The listing builds one solid part. Answer for the finished solid, in the listing's coordinates (mm). Give positions to 0.01 mm unless a question says otherwise; leave off trailing zeros. Loops run counter-clockwise (first coordinate to the right, second up) from the corner with the lowest first, then second, coordinate; pieces in that order, holes last. Notation, with made-up numbers: M 2,36.25 L 22,36.25 A21 cw 22,49.25 Z; hole C -27.75,80 d5. An arc over 180 degrees is marked long. Use one line per item in the form item = value. Start each with the question number.
1. Straight lines are drawn through the part: line 1 (X direction, y = -0.95, z = 7); line 2 (Z direction, x = -24.5, y = -0.9); line 3 (Z direction, x = -24, y = -0.8). For each, find the intervals that lie inside material, in ascending order. Write a range as from..to.
2. The part is cut by section A-A (z = 37). Write down the section's boundary in (x, y), and give its area (3 significant figures).
3. The mould has two halves that part along Z. Classify faces 1 (the face through (0, -1, -30)), 2 (the face through (-23.265, -0.986, 6.772)), 3 (the face through (32, -1, 23)): released by +Z, released by -Z, zero draft, split by the parting line, or undercut.
4. The part is cut by section B-B (z = 67). Write down the section's boundary in (x, y).
from build123d import *

# Parameters (mm, degrees)
SKETCH1_W          = 64
SKETCH1_H          = 2
BASE_FLANGE1_DEPTH = 74
SKETCH2_R          = 1.75
CUT_EXTRUDE1_DEPTH = 10
CHAMFER1_SIZE      = 2
SKETCH8_W          = 64
SKETCH8_H          = 30
TAB1_DEPTH         = 2
CHAMFER2_SIZE      = 2
CUT_EXTRUDE2_REACH = 82.647
SKETCH9_R          = 2.25


# Sheet-metal steps are written as plain solids
with BuildPart() as part:
    # Sketch1 → Base-Flange1 (new body)
    with BuildSketch(Plane.XY):
        with Locations((0, -1)):
            Rectangle(SKETCH1_W, SKETCH1_H)
    extrude(amount=BASE_FLANGE1_DEPTH)

    # Sketch2 → Cut-Extrude1 (cut)
    with BuildSketch(Plane(origin=(0, 0, 0), x_dir=(1, 0, 0), z_dir=(0, 1, 0))):
        with Locations(Location((-25, -7, 0), (0, 0, 270))):
            Circle(SKETCH2_R)
        with Locations(Location((-25, -67, 0), (0, 0, 270))):
            Circle(SKETCH2_R)
        with Locations(Location((25, -67, 0), (0, 0, 270))):
            Circle(SKETCH2_R)
        with Locations(Location((25, -7, 0), (0, 0, 270))):
            Circle(SKETCH2_R)
    extrude(amount=-CUT_EXTRUDE1_DEPTH, mode=Mode.SUBTRACT)

    # Chamfer1
    chamfer1_edges = [part.edges().sort_by_distance(p)[0] for p in [
        (-32, -1, 74),
        (32, -1, 74),
    ]]
    chamfer(chamfer1_edges, length=CHAMFER1_SIZE)

    # Sketch8 → Tab1 (add)
    with BuildSketch(Plane(origin=(0, 0, 0), x_dir=(1, 0, 0), z_dir=(0, 1, 0))):
        with Locations((0, 15)):
            Rectangle(SKETCH8_W, SKETCH8_H)
    extrude(amount=-TAB1_DEPTH)

    # Chamfer2
    chamfer2_edges = [part.edges().sort_by_distance(p)[0] for p in [
        (-32, -1, -30),
        (32, -1, -30),
    ]]
    chamfer(chamfer2_edges, length=CHAMFER2_SIZE)

    # Sketch9 → Cut-Extrude2 (cut, up to next)
    with BuildSketch(Plane(origin=(0, 0, 0), x_dir=(1, 0, 0), z_dir=(0, 1, 0)), mode=Mode.PRIVATE) as cut_extrude2_sk1:
        with Locations(Location((-25.25, -37, 0), (0, 0, 270))):
            Circle(SKETCH9_R)
    cut_extrude2_tool1 = extrude(cut_extrude2_sk1.sketch, amount=-CUT_EXTRUDE2_REACH, mode=Mode.PRIVATE) & part.part
    # Sketch9 → Cut-Extrude2 (cut, up to next)
    with BuildSketch(Plane(origin=(0, 0, 0), x_dir=(1, 0, 0), z_dir=(0, 1, 0)), mode=Mode.PRIVATE) as cut_extrude2_sk2:
        with Locations(Location((25.25, -37, 0), (0, 0, 270))):
            Circle(SKETCH9_R)
    cut_extrude2_tool2 = extrude(cut_extrude2_sk2.sketch, amount=-CUT_EXTRUDE2_REACH, mode=Mode.PRIVATE) & part.part
    add(cut_extrude2_tool1.solids().sort_by_distance((-25.25, 0, 37))[0], mode=Mode.SUBTRACT)
    add(cut_extrude2_tool2.solids().sort_by_distance((25.25, 0, 37))[0], mode=Mode.SUBTRACT)


solid = part.part
Derived:
q1.line_1 = -32..-26.75, -23.25..23.25, 26.75..32
q1.line_2 = -30..5.32, 8.68..34.88, 39.12..65.32, 68.68..74
q1.line_3 = -30..5.56, 8.44..35.13, 38.87..65.56, 68.44..74
q2.outline = M -32,-2 L -27.5,-2 L -27.5,0 L -32,0 Z; M -23,-2 L 23,-2 L 23,0 L -23,0 Z; M 27.5,-2 L 32,-2 L 32,0 L 27.5,0 Z
q2.area = 110 mm2
q3.face_1 = released by -Z
q3.face_2 = undercut
q3.face_3 = zero draft
q4.outline = M -32,-2 L -26.75,-2 L -26.75,0 L -32,0 Z; M -23.25,-2 L 23.25,-2 L 23.25,0 L -23.25,0 Z; M 26.75,-2 L 32,-2 L 32,0 L 26.75,0 Z
